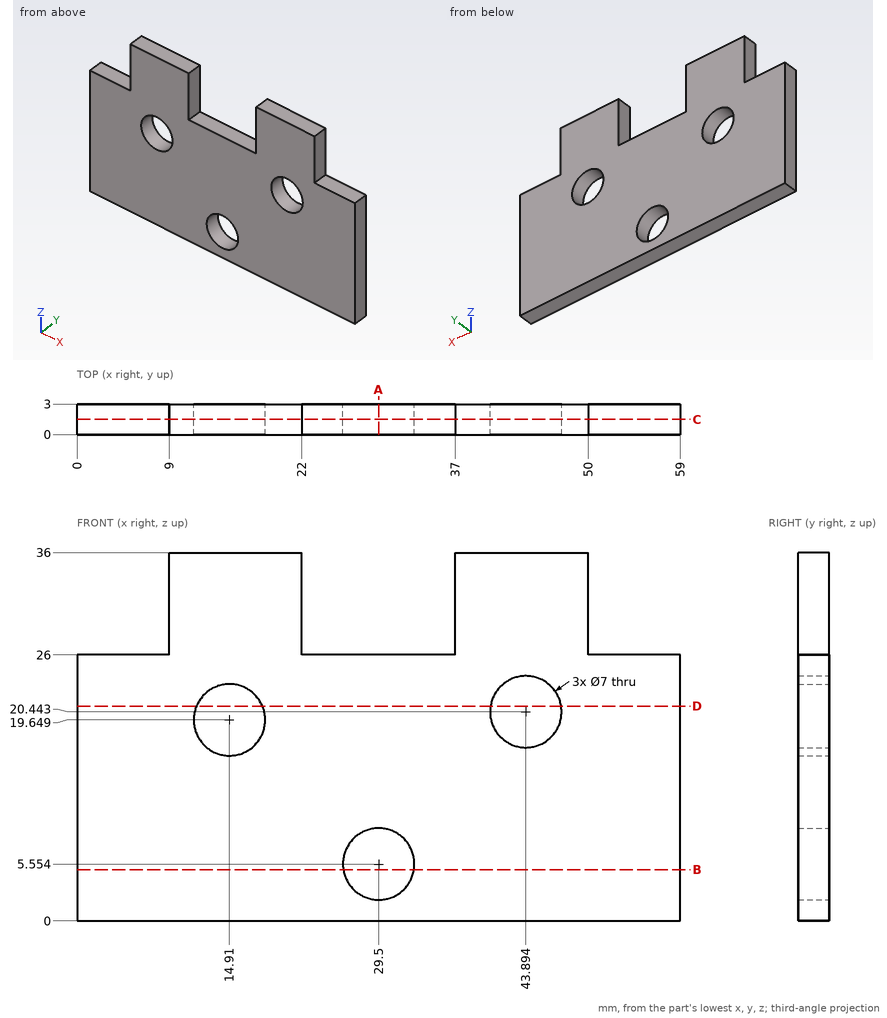
Could you check a few things on this drawing? It's one solid part, dimensions in mm from its lowest x, y, z. Round coordinates to 2 decimals unless told otherwise and drop trailing zeros. Loops run counter-clockwise (first coordinate to the right, second up) from the corner with the lowest first, then second, coordinate; pieces in that order, holes last. Notation, with made-up numbers: (-28, 47.5) -> (25, 47.5) arc R25 ccw to (25, 79.5) -> close; hole circle Ø10 at (32, 62.5). An arc over 180 degrees is marked (long way). Write each question's results on one line, items separated by ' | '.
(1) If we section it at D-D, the plane z = 21: List the corners of the cut face in (x, y) for me, then the cut area to 3 significant figures.
Worked answers:
outline: (0, 0) -> (11.68, 0) -> (11.68, 3) -> (0, 3) -> close; (18.14, 0) -> (40.44, 0) -> (40.44, 3) -> (18.14, 3) -> close; (47.35, 0) -> (59, 0) -> (59, 3) -> (47.35, 3) -> close | area: 137 mm2
(2) For P1, Ø1.5, axis at x = 26, y = 0.5, coming from the +Z side; P2, Ø0.9, axis at y = 2, z = 31, coming from the +X side; P3, Ø1.5, axis at y = 1.5, z = 29, coming from the -X side, each with a flat end and sliding along its axis, tell me the tip position at first contact or that it passes through.
Worked answers:
P1: z = 26 | P2: x = 50 | P3: x = 9
(3) If we section it at A-A, the plane x = 29.5: List the corners of the cut face in (y, z) for me (1 decimal).
Worked answers:
outline: (0, 0) -> (3, 0) -> (3, 2.1) -> (0, 2.1) -> close; (0, 9.1) -> (3, 9.1) -> (3, 26) -> (0, 26) -> close
(4) If I drill on L1, parallel to Z at x = 29.5, y = 1.3 (1 decimal); L2, parallel to X at y = 1.1, z = 21; L3, parallel to X at y = 2.55, z = 22 (1 decimal), over which ranges is the centre line in solid material (lowest first)?
Worked answers:
L1: 0 to 2.1, 9.1 to 26 | L2: 0 to 11.68, 18.14 to 40.44, 47.35 to 59 | L3: 0 to 12.3, 17.5 to 40.8, 47 to 59
(5) If we section it at B-B, the plane z = 5: List the corners of the cut face in (x, y) for me (1 decimal).
Worked answers:
outline: (0, 0) -> (26, 0) -> (26, 3) -> (0, 3) -> close; (33, 0) -> (59, 0) -> (59, 3) -> (33, 3) -> close
(6) If we section it at C-C, the plane y = 1.5: Give the number of separate pieces and of enclosed holes in the cut face, then the cut area to 3 significant figures.
Worked answers:
separate pieces: 1 | enclosed holes: 3 | area: 1,680 mm2
